```python
from build123d import *

# Parameters (mm, degrees)
BOSS_EXTRUDE1_DEPTH          = 15
SKETCH6_R                    = 3
SKETCH6_R_2                  = 1.8288
HUB_MOUNT_HOLE_PATTERN_DEPTH = 62.660360038
SKETCH7_R                    = 1.75
SKETCH7_R_2                  = 3.25
MOTOR_HOLE_PATTERN_DEPTH     = 62.660360038
SKETCH8_R                    = 18.75
MOTOR_CUTOUT_DEPTH           = 5
HUB_START                    = -7
HUB_MOUNT_CUTOUT_DEPTH       = 7
SKETCH10_R                   = 5
BOSS_EXTRUDE2_DEPTH          = 5.5
LINKAGE_PIN_HOLE_DEPTH       = 62.660360038
LINKAGE_PIN_HOLE_DEPTH_BACK  = 62.660360038
SKETCH12_R                   = 1.55
CHAMFER1_SIZE                = 2.75
SKETCH13_R                   = 6.1
CUT_EXTRUDE7_DEPTH           = 7.1
SKETCH14_R                   = 6.5
CUT_EXTRUDE8_DEPTH           = 3
SKETCH15_R                   = 3.5
CUT_EXTRUDE9_DEPTH           = 5
CUT_EXTRUDE10_DEPTH          = 62.312722986
CUT_EXTRUDE10_DEPTH_BACK     = 3
SKETCH16_R                   = 3
CUT_EXTRUDE12_DEPTH          = 7
BOSS_EXTRUDE3_REACH          = 63.784
CUT_EXTRUDE13_DEPTH          = 62.660360038
CUT_EXTRUDE13_DEPTH_BACK     = 3
SKETCH19_R                   = 4
FILLET1_R                    = 5


with BuildPart() as part:
    # Sketch2 → Boss-Extrude1 (new body)
    with BuildSketch(Plane.XY):
        with BuildLine():
            Line((-2.971428571, 12.655852885), (30.2, 20.444070045))
            ThreePointArc((30.2, 20.444070045), (56, 0), (30.2, -20.444070045))
            Line((30.2, -20.444070045), (-2.971428571, -12.655852885))
            ThreePointArc((-2.971428571, -12.655852885), (-13, 0), (-2.971428571, 12.655852885))
        make_face()
    extrude(amount=BOSS_EXTRUDE1_DEPTH)

    # Sketch6 → hub mount hole pattern (cut, through all)
    with BuildSketch(Plane.XY.offset(15)):
        Circle(SKETCH6_R)
        with Locations((-6.914797213, 6.914797213)):
            Circle(SKETCH6_R_2)
        with Locations((6.914797213, 6.914797213)):
            Circle(SKETCH6_R_2)
        with Locations((6.914797213, -6.914797213)):
            Circle(SKETCH6_R_2)
        with Locations((-6.914797213, -6.914797213)):
            Circle(SKETCH6_R_2)
    extrude(amount=-HUB_MOUNT_HOLE_PATTERN_DEPTH, mode=Mode.SUBTRACT)

    # Sketch7 → motor hole pattern (cut, through all)
    with BuildSketch(Plane.XY.offset(15)):
        with Locations((21.576606241, 7.75)):
            Circle(SKETCH7_R)
        with Locations((35, 15.5)):
            Circle(SKETCH7_R)
        with Locations((48.423393759, 7.75)):
            Circle(SKETCH7_R)
        with Locations((48.423393759, -7.75)):
            Circle(SKETCH7_R)
        with Locations((35, -15.5)):
            Circle(SKETCH7_R)
        with Locations((21.576606241, -7.75)):
            Circle(SKETCH7_R)
        with Locations((42, 0)):
            Circle(SKETCH7_R_2)
    extrude(amount=-MOTOR_HOLE_PATTERN_DEPTH, mode=Mode.SUBTRACT)

    # Sketch8 → motor cutout (cut)
    with BuildSketch(Plane.XY.offset(15)):
        with Locations((35, 0)):
            Circle(SKETCH8_R)
    extrude(amount=-MOTOR_CUTOUT_DEPTH, mode=Mode.SUBTRACT)

    # Sketch9 → hub mount cutout (cut)
    with BuildSketch(Plane.XY.offset(15).offset(HUB_START)):
        with BuildLine():
            ThreePointArc((-7.281143007, 10.769631215), (-13, 0), (-7.281143007, -10.769631215))
            ThreePointArc((-7.281143007, -10.769631215), (-6.15529138, -10.711783559), (-5.093815501, -10.332103173))
            ThreePointArc((-5.093815501, -10.332103173), (-4.17580433, -10.057753531), (-3.223255475, -10.161014917))
            ThreePointArc((-3.223255475, -10.161014917), (0, -10.66), (3.223255475, -10.161014917))
            ThreePointArc((3.223255475, -10.161014917), (4.17580433, -10.057753531), (5.093815501, -10.332103173))
            ThreePointArc((5.093815501, -10.332103173), (9.652858062, -9.652858062), (10.332103173, -5.093815501))
            ThreePointArc((10.332103173, -5.093815501), (10.057753531, -4.17580433), (10.161014917, -3.223255475))
            ThreePointArc((10.161014917, -3.223255475), (10.66, 0), (10.161014917, 3.223255475))
            ThreePointArc((10.161014917, 3.223255475), (10.057753531, 4.17580433), (10.332103173, 5.093815501))
            ThreePointArc((10.332103173, 5.093815501), (9.652858062, 9.652858062), (5.093815501, 10.332103173))
            ThreePointArc((5.093815501, 10.332103173), (4.17580433, 10.057753531), (3.223255475, 10.161014917))
            ThreePointArc((3.223255475, 10.161014917), (0, 10.66), (-3.223255475, 10.161014917))
            ThreePointArc((-3.223255475, 10.161014917), (-4.17580433, 10.057753531), (-5.093815501, 10.332103173))
            ThreePointArc((-5.093815501, 10.332103173), (-6.15529138, 10.711783559), (-7.281143007, 10.769631215))
        make_face()
    extrude(amount=HUB_MOUNT_CUTOUT_DEPTH, mode=Mode.SUBTRACT)

    # Sketch10 → Boss-Extrude2 (add)
    with BuildSketch(Plane(origin=(0, 0, 0), x_dir=(-1, 0, 0), z_dir=(0, 0, -1))):
        with Locations(Location((-11, 0, 0), (0, 0, 180))):
            Circle(SKETCH10_R)
    extrude(amount=BOSS_EXTRUDE2_DEPTH)

    # Sketch12 → Linkage pin hole (cut, two sides: drawn at the far end of the back side and taken through both)
    with BuildSketch(Plane.XY.offset(-LINKAGE_PIN_HOLE_DEPTH_BACK)):
        with Locations((11, 0)):
            Circle(SKETCH12_R)
    extrude(amount=LINKAGE_PIN_HOLE_DEPTH + LINKAGE_PIN_HOLE_DEPTH_BACK, mode=Mode.SUBTRACT)

    # Chamfer1
    chamfer1_edges = [part.edges().sort_by_distance(p)[0] for p in [
        (6, 0, -5.5),
    ]]
    chamfer(chamfer1_edges, length=CHAMFER1_SIZE)

    # Sketch13 → Cut-Extrude7 (cut)
    with BuildSketch(Plane.XY.offset(10)):
        with Locations((42, 0)):
            Circle(SKETCH13_R)
    extrude(amount=-CUT_EXTRUDE7_DEPTH, mode=Mode.SUBTRACT)

    # Sketch14 → Cut-Extrude8 (cut)
    with BuildSketch(Plane.XY.offset(8)):
        Circle(SKETCH14_R)
    extrude(amount=-CUT_EXTRUDE8_DEPTH, mode=Mode.SUBTRACT)

    # Sketch15 → Cut-Extrude9 (cut)
    with BuildSketch(Plane(origin=(0, 0, 0), x_dir=(-1, 0, 0), z_dir=(0, 0, -1))):
        with Locations((-21.576606241, -7.75)):
            Circle(SKETCH15_R)
        with Locations((-35, -15.5)):
            Circle(SKETCH15_R)
        with Locations((-48.423393759, -7.75)):
            Circle(SKETCH15_R)
        with Locations((-48.423393759, 7.75)):
            Circle(SKETCH15_R)
        with Locations((-35, 15.5)):
            Circle(SKETCH15_R)
        with Locations((-21.576606241, 7.75)):
            Circle(SKETCH15_R)
    extrude(amount=-CUT_EXTRUDE9_DEPTH, mode=Mode.SUBTRACT)

    # Sketch16 → Cut-Extrude10 (cut, two sides: drawn at the far end of the back side and taken through both)
    with BuildSketch(Plane.XY.offset(8).offset(-CUT_EXTRUDE10_DEPTH_BACK)):
        with Locations(Location((11, 0, 0), (0, 0, 104.35596801))):
            Circle(SKETCH16_R)
    extrude(amount=CUT_EXTRUDE10_DEPTH + CUT_EXTRUDE10_DEPTH_BACK, mode=Mode.SUBTRACT)

    # Sketch17 → Cut-Extrude12 (cut)
    with BuildSketch(Plane.XY.offset(10)):
        with BuildLine():
            ThreePointArc((39.857142857, 8.741176309), (25, 0), (39.857142857, -8.741176309))
            ThreePointArc((39.857142857, -8.741176309), (33, 0), (39.857142857, 8.741176309))
        make_face()
    extrude(amount=-CUT_EXTRUDE12_DEPTH, mode=Mode.SUBTRACT)

    # Sketch18 → Boss-Extrude3 (add, up to next)
    with BuildSketch(Plane.XY.offset(10), mode=Mode.PRIVATE) as boss_extrude3_sk1:
        with BuildLine():
            Line((27.471985333, -6.582476371), (33.992343948, -4.108216712))
            ThreePointArc((33.992343948, -4.108216712), (33.585458911, -3.193039032), (33.282779719, -2.238318693))
            Line((33.282779719, -2.238318693), (26.280269544, -4.895538864))
            ThreePointArc((26.280269544, -4.895538864), (26.83245784, -5.769857456), (27.471985333, -6.582476371))
        make_face()
    boss_extrude3_tool1 = extrude(boss_extrude3_sk1.sketch, amount=-BOSS_EXTRUDE3_REACH, mode=Mode.PRIVATE) - part.part
    # Sketch18 → Boss-Extrude3 (add, up to next)
    with BuildSketch(Plane.XY.offset(10), mode=Mode.PRIVATE) as boss_extrude3_sk2:
        with BuildLine():
            Line((27.471985333, 6.582476371), (33.992343948, 4.108216712))
            ThreePointArc((33.992343948, 4.108216712), (33.585458911, 3.193039032), (33.282779719, 2.238318693))
            Line((33.282779719, 2.238318693), (26.280269544, 4.895538864))
            ThreePointArc((26.280269544, 4.895538864), (26.83245784, 5.769857456), (27.471985333, 6.582476371))
        make_face()
    boss_extrude3_tool2 = extrude(boss_extrude3_sk2.sketch, amount=-BOSS_EXTRUDE3_REACH, mode=Mode.PRIVATE) - part.part
    add(boss_extrude3_tool1.solids().sort_by_distance((30.216616, -4.45872, 10))[0])
    add(boss_extrude3_tool2.solids().sort_by_distance((30.216616, 4.45872, 10))[0])

    # Sketch19 → Cut-Extrude13 (cut, two sides: drawn at the far end of the back side and taken through both)
    with BuildSketch(Plane(origin=(0, 0, 0), x_dir=(-1, 0, 0), z_dir=(0, 0, -1)).offset(-CUT_EXTRUDE13_DEPTH_BACK)):
        with Locations(Location((-6.914797213, -6.914797213, 0), (0, 0, 90.325769881))):
            Circle(SKETCH19_R)
        with Locations(Location((-6.914797213, 6.914797213, 0), (0, 0, 269.674230119))):
            Circle(SKETCH19_R)
        with Locations((6.914797213, 6.914797213)):
            Circle(SKETCH19_R)
        with Locations((6.914797213, -6.914797213)):
            Circle(SKETCH19_R)
    extrude(amount=CUT_EXTRUDE13_DEPTH + CUT_EXTRUDE13_DEPTH_BACK, mode=Mode.SUBTRACT)

    # Fillet1
    # the kernel refuses this fillet: 5 mm, written as the material it adds along each edge
    with BuildSketch(Plane(origin=(11, 0, 0), x_dir=(-0.9999950652018581, 0.003141587485879405, 0), z_dir=(-0.003141587485879405, -0.9999950652018581, 0))) as fillet1_piece_1_section:
        with BuildLine():
            CenterArc((9.465142775, 5), FILLET1_R, 206.74368395, 63.25631605)
            Line((9.465142775, 0), (9.465142775, -0.1))
            Line((9.465142775, -0.1), (5, -0.1))
            Line((5, -0.1), (4.9, 0))
            ThreePointArc((4.9, 0), (4.9, 1.375), (4.910697145, 2.705))
            Line((4.910697145, 2.705), (5, 2.75))
        make_face()
    fillet1_piece_1 = revolve(axis=Axis((11, 0, 0), (0, 0, -1)), revolution_arc=359.64, mode=Mode.PRIVATE)
    fillet1_piece_1 = fillet1_piece_1 - Plane(origin=(6.914797213, -6.914797213, -0.762875984), x_dir=(0.0056857263926290095, 0.9999838361270588, 0), z_dir=(0, 0, 1)) * Cylinder(4, 38, mode=Mode.PRIVATE)
    fillet1_piece_1 = fillet1_piece_1 - Plane(origin=(6.914797213, 6.914797213, -0.762875984), x_dir=(0.00568572639262881, -0.9999838361270588, 0), z_dir=(0, 0, 1)) * Cylinder(4, 38, mode=Mode.PRIVATE)
    fillet1_piece_1 = fillet1_piece_1 - Plane(origin=(0, 0, -0.762875984), x_dir=(1, 0, 0), z_dir=(0, 0, 1)) * Cylinder(3, 38, mode=Mode.PRIVATE)
    add(fillet1_piece_1)
    with BuildSketch(Plane(origin=(11, 0, 0), x_dir=(0.9593586032510993, -0.2821897772211103, 0), z_dir=(0.2821897772211103, 0.9593586032510993, 0))) as fillet1_piece_2_section:
        with BuildLine():
            CenterArc((9.465142775, 5), FILLET1_R, 206.74368395, 63.25631605)
            Line((9.465142775, 0), (9.465142775, -0.1))
            Line((9.465142775, -0.1), (5, -0.1))
            Line((5, -0.1), (4.9, 0))
            ThreePointArc((4.9, 0), (4.9, 1.375), (4.910697145, 2.705))
            Line((4.910697145, 2.705), (5, 2.75))
        make_face()
    fillet1_piece_2 = revolve(axis=Axis((11, 0, 0), (0, 0, -1)), revolution_arc=327.218117947, mode=Mode.PRIVATE)
    fillet1_piece_2 = fillet1_piece_2 - Plane(origin=(6.914797213, -6.914797213, -0.749324739), x_dir=(0.0056857263926290095, 0.9999838361270588, 0), z_dir=(0, 0, 1)) * Cylinder(4, 38, mode=Mode.PRIVATE)
    fillet1_piece_2 = fillet1_piece_2 - Plane(origin=(6.914797213, 6.914797213, -0.749324739), x_dir=(0.00568572639262881, -0.9999838361270588, 0), z_dir=(0, 0, 1)) * Cylinder(4, 38, mode=Mode.PRIVATE)
    fillet1_piece_2 = fillet1_piece_2 - Plane(origin=(0, 0, -0.749324739), x_dir=(1, 0, 0), z_dir=(0, 0, 1)) * Cylinder(3, 38, mode=Mode.PRIVATE)
    add(fillet1_piece_2)


solid = part.part
```
For this review, take the finished solid that the model builds, in its own axes (mm). A direction names the side the tool comes from. Round coordinates to 2 decimals unless told otherwise and drop trailing zeros. Write each loop counter-clockwise with the first axis right and the second up, starting at its lowest first coordinate (ties: lowest second). Pieces come first, ordered by that corner, then holes.
1) Machinability: for faces 1 (the face through (10.057, 4.162, 11.451)), 2 (the face through (8.47, 3.23, 1.18)), 3 (the face through (34, 8, 3)), which of the approach directions +Z, -Z, +X, -X, +Y, -Y give a long, thin tool a straight path to every point of the face, cutting with its end or side? Answer none if there is none.
Answer below:
face 1: +Z, -X
face 2: -Z
face 3: +Z
2) Insertion check: pin 1 Ø12 at (x, y) = (3.5, -10) entering from +Z; pin 2 Ø2 at (x, y) = (23, 9) entering from -Z; pin 3 Ø4 at (x, y) = (-6.91, 6.91) entering from +Z; pin 4 Ø10 at (x, y) = (40, 4) entering from -Z. Each pin has a flat end and moves straight along its axis. Give the tip position at first contact, or say it passes through.
Answer below:
pin 1: stops at z = 15
pin 2: stops at z = 5
pin 3: stops at z = 8
pin 4: stops at z = 0
3) For line 1 along Y through (x, z) = (35, 1.85); line 2 along Y through (x, z) = (21, 9.5); line 3 along Z through (x, y) = (19.5, -6), list the stretches that pass through material, from the lowest coordinate up.
Answer below:
line 1: y = -21 to -19, -12 to 12, 19 to 21
line 2: y = -18.28 to -9.4, -6.1 to 6.1, 9.4 to 18.28
line 3: z = 5 to 10
4) Take a section at B-B on y = -15.5. Give the boundary of the cut face in (x, z), then the cut area to 3 significant figures.
Answer below:
outline: (9.14, 0) - (31.5, 0) - (31.5, 5) - (33.25, 5) - (33.25, 10) - (24.45, 10) - (24.45, 15) - (9.14, 15) - close; (36.75, 5) - (38.5, 5) - (38.5, 0) - (49.17, 0) - (49.17, 15) - (45.55, 15) - (45.55, 10) - (36.75, 10) - close
area: 442 mm2
5) Take a section at D-D on y = -7.75. State how many separate pieces and enclosed holes the cut face has, then the cut area to 3 significant figures.
Answer below:
separate pieces: 5
enclosed holes: 0
area: 412 mm2
6) Take a section at A-A on x = 41.5. Give the boundary of the cut face in (y, z).
Answer below:
outline: (-19.97, 0) - (-3.21, 0) - (-3.21, 2.9) - (-6.08, 2.9) - (-6.08, 10) - (-17.59, 10) - (-17.59, 15) - (-19.97, 15) - close; (3.21, 0) - (19.97, 0) - (19.97, 15) - (17.59, 15) - (17.59, 10) - (6.08, 10) - (6.08, 2.9) - (3.21, 2.9) - close
